```python
from build123d import *


with BuildPart() as part:
    # Sketch1 → Revolve-Thin1 (revolve)
    with BuildSketch(Plane.XY):
        Polygon((-102.279792746, 15), (-67.150259067, 15), (-67.150259067, 20), (-34.180259067, 20), (-34.180259067, 15), (85.819740933, 15), (85.819740933, 20), (118.789740933, 20), (118.789740933, 15), (175.759740933, 15), (175.759740933, 20), (208.729740933, 20), (208.729740933, 15), (218.211606218, 15), (305.314834779, 15), (305.314834779, 5), (218.211606218, 5), (198.729740933, 5), (198.729740933, 10), (185.759740933, 10), (185.759740933, 5), (108.789740933, 5), (108.789740933, 10), (95.819740933, 10), (95.819740933, 5), (-44.180259067, 5), (-44.180259067, 10), (-57.150259067, 10), (-57.150259067, 5), (-102.279792746, 5), align=None)
    revolve(axis=Axis((-102.279792746, 0, 0), (1, 0, 0)))


solid = part.part
```
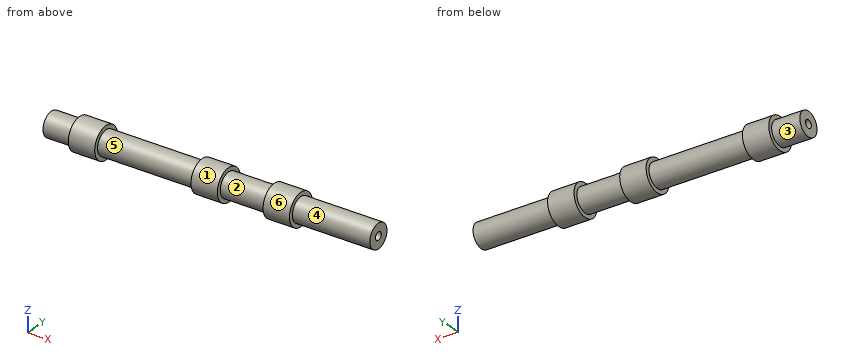
Design review of the part built by this model. Coordinates are the model's own, in mm. Face numbers are marked on the shaded views. A direction names the side the tool comes from. Round coordinates to 2 decimals unless told otherwise and drop trailing zeros. Order: outer loops, then holes, each group sorted by start corner. A loop starts at its lowest first (then second) coordinate and runs counter-clockwise, first axis right, second up. Notation, with made-up numbers: (65.25, 67) - (102.25, 67) arc R19 ccw to (102.25, 92) - close; hole circle Ø2 at (-35.75, -20.5). An arc over 180 degrees is marked (long way). One line per question, with ' | ' between items.
Item 1: For P1, Ø6, axis at x = 185, y = 16, coming from the +Z side; P2, Ø8, axis at x = 144.5, z = -5.5, coming from the +Y side; P3, Ø10, axis at x = 108.5, y = -11, coming from the +Z side; P4, Ø6, axis at y = 0, z = 0, coming from the +X side, all flat-tipped, find the tip position at first contact; note any pin that passes through.
Checks:
P1: z = 15.2 | P2: y = 14.92 | P3: z = 19.08 | P4: through
Item 2: Draft analysis for pull direction X (two halves, no side actions). For the marked faces 1 and 2, state which applies: +X half, -X half, draft (parallel to the pull), parting line (faces both ways), or undercut.
Checks:
face 1: draft | face 2: undercut
Item 3: Take a section at B-B, the plane x = 244. Write out the cut boundary in (y, z), then the cut area to 3 significant figures.
Checks:
outline: circle Ø30 at (0, 0); hole circle Ø10 at (0, 0) | area: 628 mm²
Item 4: Wall thickness on line 1 (X direction, y = 2.5, z = -6); line 2 (X direction, y = -9.5, z = 16.5); line 3 (Z direction, x = 235, y = 0): over which ranges is each line inside the solid? List them lowest first. Write a range as [from, to].
Checks:
line 1: [-102.28, -57.15], [-44.18, 95.82], [108.79, 185.76], [198.73, 305.31] | line 2: [-67.15, -34.18], [85.82, 118.79], [175.76, 208.73] | line 3: [-15, -5], [5, 15]
Item 5: Machinability: for the marked faces 3, 4, 5 and 6, which of the approach directions +Z, -Z, +X, -X, +Y, -Y give a long, thin tool a straight path to every point of the face, cutting with its end or side? Answer none if there is none.
Checks:
face 3: -X | face 4: +X | face 5: none | face 6: +X, -X
Item 6: Take a section at A-A, the plane x = -62. Write out the cut boundary in (y, z).
Checks:
outline: circle Ø40 at (0, 0); hole circle Ø10 at (0, 0)
